Geometry check sheet. Reference: the model listing, model coordinates, mm. Face numbers are marked on the shaded views. A direction names the side the tool comes from. Give positions to 0.01 mm unless a question says otherwise; leave off trailing zeros. Order: outer loops, then holes, each group sorted by start corner. A loop starts at its lowest first (then second) coordinate and runs counter-clockwise, first axis right, second up. Notation, with made-up numbers: M -38,68 L -26,68 A13 cw -26,89 Z; hole C 57,46 d4. An arc over 180 degrees is marked long. Answer as a JSON object with one key per item and string values. Group by question number.
Autodesk Inventor part; units mm, degrees
ref_plane "YZ Plane" through (0, 0, 0) normal (1, 0, 0) x (0, 1, 0)
ref_plane "XZ Plane" through (0, 0, 0) normal (0, 1, 0) x (-1, 0, 0)
ref_plane "XY Plane" through (0, 0, 0) normal (0, 0, 1) x (1, 0, 0)
sketch "Sketch1" plane through (0, 0, 0) normal (0, 0, 1) x (1, 0, 0)
  line L0 (-3.5718, -2.6632) -> (-7.5718, -2.6632)
  line L1 (-7.5718, -2.6632) -> (-7.5718, -10.8132)
  line L2 (-7.5718, -10.8132) -> (-3.5718, -10.8132)
  line L3 (-3.5718, -10.8132) -> (-3.5718, -2.6632)
  dimension "d1" = 8.15
  dimension "d2" = 4
revolve "Shoulder" add sketch "Sketch1" angle 360 about axis through (-3.5718, -10.8132, 0) along (0, 1, 0)
sketch "Sketch2" plane through (-3.5718, -2.6632, 0) normal (0, 1, 0) x (1, 0, 0)
  circle A0 centre (0, 0) radius 4
  circle A1 centre (0, 0) radius 3.76
  dimension "d3" = 7.52
extrude "Shoulder_neck" add sketch "Sketch2" along normal blind 1.85 contours A1
sketch "Sketch3" plane through (-3.5718, -0.8132, 0) normal (0, 1, 0) x (1, 0, 0)
  circle A0 centre (0, 0) radius 3.76
  circle A1 centre (0, 0) radius 6.6
  dimension "d6" = 13.2
extrude "Head" add sketch "Sketch3" along normal blind 5.5 contours A0 | A1
sketch "Sketch4" plane through (-3.5718, -10.8132, 0) normal (0, -1, 0) x (1, 0, 0)
  circle A0 centre (0, 0) radius 4
  circle A1 centre (0, 0) radius 2.255
  dimension "d9" = 4.51
extrude "Thread_neck" add sketch "Sketch4" along normal blind 2.3 contours A1
sketch "Sketch5" plane through (-3.5718, -13.1132, 0) normal (0, -1, 0) x (1, 0, 0)
  circle A0 centre (0, 0) radius 2.255
  circle A1 centre (0, 0) radius 3
  dimension "d12" = 6
extrude "Thread_shoulder" add sketch "Sketch5" along normal blind 8.7 contours A0 | A1
sketch "Sketch6" plane through (-3.5718, 4.6868, 0) normal (0, 1, 0) x (1, 0, 0)
  circle A0 centre (0, 0) radius 6.6
  circle A1 centre (0, 0) radius 2 construction
  line L0 (-2, 1.1547) -> (-2, -1.1547)
  line L1 (-2, -1.1547) -> (0, -2.3094)
  line L2 (0, -2.3094) -> (2, -1.1547)
  line L3 (2, -1.1547) -> (2, 1.1547)
  line L4 (2, 1.1547) -> (0, 2.3094)
  line L5 (0, 2.3094) -> (-2, 1.1547)
  dimension "d15" = 4
extrude "Hex" cut sketch "Sketch6" against normal blind 2.4 contours L5 L4 L3 L2 L1 L0
chamfer "Chamfer1" distance 0.24 angle 30 1 edges at (0.4282, -2.6632, 0) measured on face at (-7.4166, -2.6632, -0.619)
fillet "Fillet1" radius 0.4 1 edges at (-7.3318, -0.8132, 0)
chamfer "Chamfer2" distance 0.4 angle 30 1 edges at (-10.1718, 4.6868, 0) measured on face at (2.9427, 2.8535, 1.0587)
chamfer "Chamfer3" distance 0.4 angle 30 1 edges at (-6.5718, -21.8132, 0) measured on face at (-2.6428, -21.8132, 0.823)
fillet "Fillet2" radius 0.6 1 edges at (-5.8268, -10.8132, 0)
chamfer "Chamfer7" distance 0.745 angle 30 1 edges at (-6.5718, -13.1132, 0) measured on face at (-0.871, -13.1132, -0.4192)
thread "Thread"
equation "\"d3\" = Shoulder_neck_dia"
equation "\"d4\" = Shoulder_neck_length"
equation "\"d6\" = Head_diameter"
equation "\"d7\" = Head_height"
equation "\"d9\" = Thread_neck_dia"
equation "\"d10\" = Thread_neck_length"
equation "\"d12\" = Thread_diameter"
equation "\"d13\" = Thread_length - Thread_neck_length"
equation "\"d15\" = Hex_size"
equation "\"d16\" = Hex_length"
equation "\"d18\" = -0.5 * Shoulder_neck_dia + 0.5 * Shoulder_diameter"
equation "\"d64\" = -0.5 * Shoulder_neck_dia + 0.5 * Shoulder_diameter"
equation "\"d21\" = 0.1 * Hex_size"
equation "\"d65\" = 0.1 * Hex_size"
equation "\"d23\" = 0.5 * Thread_pitch"
equation "\"d66\" = 0.5 * Thread_pitch"
equation "\"d25\" = Thread_neck_radius"
equation "\"d60\" = -0.5 * Thread_neck_dia + 0.5 * Thread_diameter"
equation "\"d67\" = -0.5 * Thread_neck_dia + 0.5 * Thread_diameter"
equation "\"d1\" = Shoulder_length - Shoulder_neck_length"
equation "\"d2\" = 0.5 * Shoulder_diameter"
equation "\"Shoulder_diameter\" = 8"
equation "\"Shoulder_length\" = 10"
equation "\"Shoulder_neck_dia\" = 7.52"
equation "\"Thread_diameter\" = 6"
equation "\"Thread_length\" = 11"
equation "\"Head_diameter\" = 13.2"
equation "\"Head_height\" = 5.5"
equation "\"Thread_neck_dia\" = 4.51"
equation "\"Hex_size\" = 4"
equation "\"Hex_length\" = 2.4"
equation "\"Thread_pitch\" = 0.8"
equation "\"Shoulder_neck_length\" = 1.85"
equation "\"Thread_neck_length\" = 2.3"
equation "\"Thread_neck_radius\" = 0.6"
properties part number "SCREW, SHOULDER, P, 12.9, 8MMX10MM" material "Steel, High Strength Low Alloy"
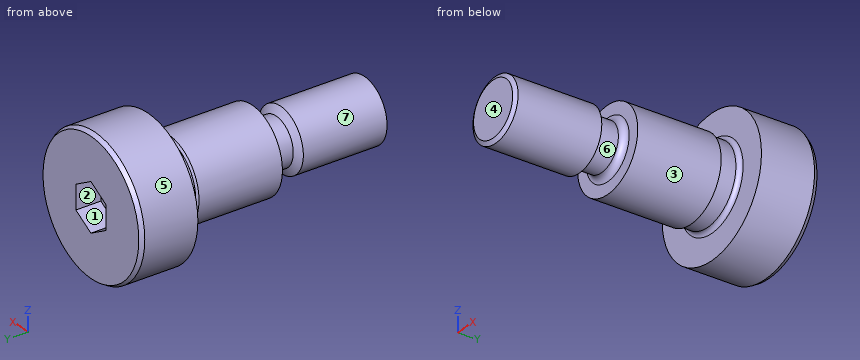
1. Cross-section at B-B (y = -10.25). Record the cut outline in (x, z), and give its area (3 significant figures).
2. Thickness scan on line 1 along Z through (x, y) = (-2.5, -18); line 2 along Y through (x, z) = (-4.5, 3.25); line 3 along Y through (x, z) = (-7.25, -2.75). Record the ranges inside material, lowest first. Write a range as [from, to].
3. Cross-section at A-A (y = -19). Record the cut outline in (x, z).
4. Depth check by flat-ended pin: pin 1 (4 mm diameter, centred on y = -18, z = 3, fed in from +X); pin 2 (1.2 mm diameter, centred on x = -4, z = 0.5, fed in from +Y); pin 3 (0.7 mm diameter, centred on y = 3.5, z = 0.5, fed in from -X). Enter the tip coordinate at first touch or a pass-through.
5. Release check for a two-part mould opening along Z. For the marked faces 1, 2, 3 and 4 record: released by +Z, released by -Z, zero draft, split by the parting line, or undercut.
6. Access from +Z, -Z, +X, -X, +Y, -Y to the whole of each face (thin tool, end or side, straight path). Record for the marked faces 5, 6 and 7.
Report:
{
 "1": {"outline": "C -3.57,0 d8", "area": "50.3 mm2"},
 "2": {"line 1": "z = [-2.8, 2.8]", "line 2": "y = [-10.81, 4.69]", "line 3": "y = [-0.81, 4.69]"},
 "3": {"outline": "C -3.57,0 d6"},
 "4": {"pin 1": "stops at x = -0.74", "pin 2": "stops at y = 2.29", "pin 3": "stops at x = -10.17"},
 "5": {"face 1": "undercut", "face 2": "undercut", "face 3": "split by the parting line", "face 4": "zero draft"},
 "6": {"face 5": "+Y, -Y", "face 6": "none", "face 7": "-Y"}
}
